from build123d import *

# Parameters (mm, degrees)
SKETCH1_W           = 42.3
SKETCH1_H           = 42.8
BOSS_EXTRUDE1_DEPTH = 3
SKETCH6_R           = 12.5
SKETCH6_R_2         = 1.6
CUT_EXTRUDE3_DEPTH  = 31.237104689
SKETCH7_W           = 42.3
SKETCH7_H           = 40.5
BOSS_EXTRUDE2_DEPTH = 3
SKETCH8_W           = 42.3
SKETCH8_H           = 4
BOSS_EXTRUDE3_DEPTH = 40
SKETCH10_R          = 2.1
CUT_EXTRUDE4_DEPTH  = 77.986573505
FILLET1_R           = 5


with BuildPart() as part:
    # Sketch1 → Boss-Extrude1 (new body)
    with BuildSketch(Plane.XY):
        Rectangle(SKETCH1_W, SKETCH1_H)
    extrude(amount=BOSS_EXTRUDE1_DEPTH)

    # Sketch6 → Cut-Extrude3 (cut, through all)
    with BuildSketch(Plane(origin=(0, 0, 0), x_dir=(-1, 0, 0), z_dir=(0, 0, -1))):
        Circle(SKETCH6_R)
        with Locations((-15.65, 15.9)):
            Circle(SKETCH6_R_2)
        with Locations((15.65, 15.9)):
            Circle(SKETCH6_R_2)
        with Locations((-15.65, -15.9)):
            Circle(SKETCH6_R_2)
        with Locations((15.65, -15.9)):
            Circle(SKETCH6_R_2)
    extrude(amount=-CUT_EXTRUDE3_DEPTH, mode=Mode.SUBTRACT)

    # Sketch7 → Boss-Extrude2 (add)
    with BuildSketch(Plane.XZ.offset(21.4)):
        with Locations((0, -17.25)):
            Rectangle(SKETCH7_W, SKETCH7_H)
    extrude(amount=BOSS_EXTRUDE2_DEPTH)

    # Sketch8 → Boss-Extrude3 (add)
    with BuildSketch(Plane.XZ.offset(24.4)):
        with Locations((0, -35.5)):
            Rectangle(SKETCH8_W, SKETCH8_H)
    extrude(amount=BOSS_EXTRUDE3_DEPTH)

    # Sketch10 → Cut-Extrude4 (cut, through all)
    with BuildSketch(Plane.XY.offset(-33.5)):
        with Locations((-12.15, -33.4)):
            Circle(SKETCH10_R)
        with Locations((12.15, -33.4)):
            Circle(SKETCH10_R)
        with Locations((-12.15, -55.4)):
            Circle(SKETCH10_R)
        with Locations((12.15, -55.4)):
            Circle(SKETCH10_R)
    extrude(amount=-CUT_EXTRUDE4_DEPTH, mode=Mode.SUBTRACT)

    # Fillet1
    fillet1_edges = [part.edges().sort_by_distance(p)[0] for p in [
        (-21.15, -64.4, -35.5),
        (21.15, -64.4, -35.5),
        (-21.15, 21.4, 1.5),
        (21.15, 21.4, 1.5),
    ]]
    fillet(fillet1_edges, radius=FILLET1_R)


solid = part.part
CAD build for the part. Positions are in the model's coordinates, mm. A direction names the side the tool comes from. Round coordinates to 2 decimals unless told otherwise and drop trailing zeros. Write each loop counter-clockwise with the first axis right and the second up, starting at its lowest first coordinate (ties: lowest second). Pieces come first, ordered by that corner, then holes. Notation, with made-up numbers: M 81,9 L 113,9 A30 cw 113,38 Z; hole C 76,64.5 d11. An arc over 180 degrees is marked long. Put each result on its own line as item: value. Start each with the question number.
1) Pin check, flat tips, straight feed: pin 1 Ø2.5 at (x, y) = (15.65, 15.9) entering from -Z; pin 2 Ø4 at (x, y) = (-8.5, -40.5) entering from +Z; pin 3 Ø11 at (x, z) = (8.5, -18.5) entering from +Y. Stop position of each tip, or through.
2) Saw through at C-C, the plane x = 7. Write the cut outline in (y, z), and give its area (3 significant figures).
3) 3-axis set-ups, long thin cutter, end or side, ignore diameter. For faces 4 (the cylindrical face through (-12.61, -57.45, -35.47)), 5 (the flat face through (-10, -9, 0)), 6 (the flat face through (0, -44, -33.5)): which of +Z, -Z, +X, -X, +Y, -Y reach the whole face in a straight line?
4) Saw through at D-D, the plane z = -2. Write the cut outline in (x, y).
5) Pull direction X, two halves, no side cores. Call faces 1 (the cylindrical face through (-17.176, -15.419, 1.479)), 2 (the flat face through (9, 9, 3)), 3 (the cylindrical face through (19.65, -62.97, -35.47)): pulls with the +X half, pulls with the -X half, needs draft (parallel to the pull), parting line crosses it, or undercut.
6) Saw through at A-A, the plane y = 0. Write the cut outline in (x, z), and give its area (3 significant figures).
7) Saw through at B-B, the plane y = -33.4. Write the cut outline in (x, z), and give its area (3 significant figures).
8) Drill centre lines: probe 1 along Y at (x, z) = (12.15, -34.55); probe 2 along Y at (x, z) = (15.65, 2.25); probe 3 along X at (y, z) = (-33, -35). Where is each one in solid material? Low to high. Write a range as [from, to].
Resolved:
1. pin 1: through
1. pin 2: z = -33.5
1. pin 3: y = -21.4
2. outline: M -64.4,-37.5 L -21.4,-37.5 L -21.4,0 L -10.36,0 L -10.36,3 L -24.4,3 L -24.4,-33.5 L -64.4,-33.5 Z; M 10.36,0 L 21.4,0 L 21.4,3 L 10.36,3 Z
2. area: 348 mm²
3. face 4: +Z, -Z
3. face 5: -Z, +X, -X, +Y
3. face 6: +Z, +X, -X, -Y
4. outline: M -21.15,-24.4 L 21.15,-24.4 L 21.15,-21.4 L -21.15,-21.4 Z
5. face 1: undercut
5. face 2: needs draft
5. face 3: pulls with the +X half
6. outline: M -21.15,0 L -12.5,0 L -12.5,3 L -21.15,3 Z; M 12.5,0 L 21.15,0 L 21.15,3 L 12.5,3 Z
6. area: 51.9 mm²
7. outline: M -21.15,-37.5 L -14.25,-37.5 L -14.25,-33.5 L -21.15,-33.5 Z; M -10.05,-37.5 L 10.05,-37.5 L 10.05,-33.5 L -10.05,-33.5 Z; M 14.25,-37.5 L 21.15,-37.5 L 21.15,-33.5 L 14.25,-33.5 Z
7. area: 136 mm²
8. probe 1: [-64.4, -57.5], [-53.3, -35.5], [-31.3, -21.4]
8. probe 2: [-24.4, -17.5], [-14.3, 14.3], [17.5, 21.4]
8. probe 3: [-21.15, -14.21], [-10.09, 10.09], [14.21, 21.15]
